Source: CAD feature listing. Evaluate the final solid. Frame: model axes, mm. A direction names the side the tool comes from. Round coordinates to 2 decimals unless told otherwise and drop trailing zeros. Write item = value, one per line. Start each with the question number.
from build123d import *

# Parameters (mm, degrees)
SKETCH027_R          = 38.1
PAD009_DEPTH         = 22.5
POCKET015_DEPTH      = 278.563668
POCKET015_DEPTH_BACK = -233.563668
POLARPATTERN_COUNT   = 8
SKETCH029_R          = 1.6
POCKET016_DEPTH      = 45.001
POCKET016_DEPTH_BACK = -0.001
SKETCH030_R          = 32.1
POCKET017_DEPTH      = 1
SKETCH031_R          = 12
POCKET018_DEPTH      = 19
SKETCH034_R          = 32.1
POCKET019_DEPTH      = 1
SKETCH035_R          = 8
POCKET020_DEPTH      = 13
SKETCH069_R          = 1.6
POCKET040_DEPTH      = 8


with BuildPart() as part:
    # Sketch027 → Pad009 (new body, symmetric)
    with BuildSketch(Plane.YZ):
        Circle(SKETCH027_R)
    extrude(amount=PAD009_DEPTH, both=True)

    # Sketch028 (on Face3 of Pad009) → Pocket015 (cut, two sides)
    with BuildSketch(Plane.YZ.offset(22.5)) as pocket015_sk:
        with BuildLine():
            ThreePointArc((1.865103, 9.926298), (0, 10.1), (-1.865103, 9.926298))
            Line((-1.865103, 9.926298), (-8.518771, 28.86937))
            ThreePointArc((8.518771, 28.86937), (0, 30.1), (-8.518771, 28.86937))
            Line((8.518771, 28.86937), (1.865103, 9.926298))
        make_face()
    pocket015 = extrude(amount=-POCKET015_DEPTH, mode=Mode.SUBTRACT)
    extrude(pocket015_sk.sketch, amount=-POCKET015_DEPTH_BACK, mode=Mode.SUBTRACT)

    # PolarPattern: Pocket015 ×8 about axis
    polarpattern_axis = Axis((22.5, 0, 0), (1, 0, 0))
    for i in range(1, POLARPATTERN_COUNT):
        add(pocket015.rotate(polarpattern_axis, i * 360 / POLARPATTERN_COUNT), mode=Mode.SUBTRACT)

    # Sketch029 (on Face3 of PolarPattern) → Pocket016 (cut, two sides)
    with BuildSketch(Plane.YZ.offset(22.5)) as pocket016_sk:
        Circle(SKETCH029_R)
    extrude(amount=-POCKET016_DEPTH, mode=Mode.SUBTRACT)
    extrude(pocket016_sk.sketch, amount=-POCKET016_DEPTH_BACK, mode=Mode.SUBTRACT)

    # Sketch030 (on Face2 of Pocket016) → Pocket017 (cut)
    with BuildSketch(Plane(origin=(-22.5, 0, 0), x_dir=(0, 1, 0), z_dir=(-1, 0, 0))):
        Circle(SKETCH030_R)
    extrude(amount=-POCKET017_DEPTH, mode=Mode.SUBTRACT)

    # Sketch031 (on Face38 of Pocket017) → Pocket018 (cut)
    with BuildSketch(Plane(origin=(-21.5, 0, 0), x_dir=(0, 1, 0), z_dir=(-1, 0, 0))):
        Circle(SKETCH031_R)
    extrude(amount=-POCKET018_DEPTH, mode=Mode.SUBTRACT)

    # Sketch033 → Groove (revolve, cut)
    with BuildSketch(Plane.XZ):
        Polygon((-16.5, 38.1), (16.5, 38.1), (16.5, 36.1), (18.5, 36.1), (18.5, 34.1), (-18.5, 34.1), (-18.5, 36.1), (-16.5, 36.1), align=None)
    revolve(axis=Axis((0, 0, 0), (1, 0, 0)), mode=Mode.SUBTRACT)

    # Sketch034 (on Face41 of Groove) → Pocket019 (cut)
    with BuildSketch(Plane.YZ.offset(22.5)):
        Circle(SKETCH034_R)
    extrude(amount=-POCKET019_DEPTH, mode=Mode.SUBTRACT)

    # Sketch035 (on Face41 of Pocket019) → Pocket020 (cut)
    with BuildSketch(Plane.YZ.offset(21.5)):
        Circle(SKETCH035_R)
    extrude(amount=-POCKET020_DEPTH, mode=Mode.SUBTRACT)

    # Cone → Cone (revolve, cut)
    with BuildSketch(Plane(origin=(8.086737, 0, 0), x_dir=(0, 1, 0), z_dir=(0, 0, -1))):
        Polygon((0, 0), (12, 0), (31, 14), (0, 14), align=None)
    revolve(axis=Axis((8.086737, 0, 0), (1, 0, 0)), mode=Mode.SUBTRACT)

    # Cone001 → Cone001 (revolve, cut)
    with BuildSketch(Plane(origin=(-2.5, 0, 0), x_dir=(0, 1, 0), z_dir=(0, 0, 1))):
        Polygon((0, 0), (12, 0), (30, 19), (0, 19), align=None)
    revolve(axis=Axis((-2.5, 0, 0), (-1, 0, 0)), mode=Mode.SUBTRACT)

    # Sketch069 (on Face42 of Cone001) → Pocket040 (cut)
    with BuildSketch(Plane(origin=(-2.5, 0, 0), x_dir=(0, 1, 0), z_dir=(-1, 0, 0))):
        with Locations((-7.071068, 0)):
            Circle(SKETCH069_R)
        with Locations((0, 7.071068)):
            Circle(SKETCH069_R)
        with Locations((7.071068, 0)):
            Circle(SKETCH069_R)
        with Locations((0, -7.071068)):
            Circle(SKETCH069_R)
    extrude(amount=-POCKET040_DEPTH, mode=Mode.SUBTRACT)


with BuildPart() as part_1:
    # Body006 placement: moved
    add(part.part.moved(Location((7.1, 0, 0))))


solid = part_1.part
(1) Pin query (flat end, axial travel): P1, Ø4, axis at y = 0, z = -7.07, coming from the +X side; P2, Ø2, axis at x = 2, z = -21.5, coming from the -Y side; P3, Ø2.5, axis at y = 7.5, z = -0.5, coming from the -X side; P4, Ø3, axis at y = 0, z = 0, coming from the -X side. Return the tip coordinate at first contact, or that it passes through.
(2) Mould query, pull axis Z, two halves, no side actions, for faces 1 (the face through (7.36, 21.37, 21.2)), 2 (the face through (-9.4, 34, -14)). Classes: +Z half, -Z half, draft (parallel to the pull), parting line (faces both ways), or undercut.
(3) Material intervals for line 1 along Z through (x, y) = (8, 0); line 2 along X through (y, z) = (31.5, -19.5); line 3 along Z through (x, y) = (-15, 0), sorted ascending. Write a range as from..to.
(4) Cut plane B-B (y = 0). State how many separate pieces and enclosed holes the cut face has, and give its area (3 significant figures).
(5) Access query for faces 3 (the face through (7.362, 19.525, 11.071)), 4 (the face through (23.6, 14, 34)), 5 (the face through (29.1, -25.5, -19.5)), 6 (the face through (12.6, 0, -7)). Directions: +Z, -Z, +X, -X, +Y, -Y. A direction counts if a zero-diameter tool reaches every point of the face in a straight line with its end or side. Return the directions, or none.
Solution:
q1.P1 = 15.19
q1.P2 = -27.25
q1.P3 = 4.6
q1.P4 = through
q2.face_1 = undercut
q2.face_2 = draft
q3.line_1 = -34.1..-30.1, -10.1..-8.67, -5.47..-1.6, 1.6..5.47, 8.67..10.1, 30.1..34.1
q3.line_2 = -15.4..-9.4, 23.6..29.6
q3.line_3 = -38.1..-32.1, 32.1..38.1
q4.separate_pieces = 4
q4.enclosed_holes = 0
q4.area = 561 mm^2
q5.face_3 = +X, -X
q5.face_4 = none
q5.face_5 = +X
q5.face_6 = -X
